Geometry check sheet. Reference: the model listing, model coordinates, mm. A direction names the side the tool comes from. Coordinates: 2 decimals unless noted, no trailing zeros. Loops run counter-clockwise (first coordinate to the right, second up) from the corner with the lowest first, then second, coordinate; pieces in that order, holes last. Notation, with made-up numbers: (-33.75, -10) -> (-19.75, -10) arc R18 ccw to (-19.75, 8) -> close; hole circle Ø11 at (-15, -10.5). An arc over 180 degrees is marked (long way). Answer as a JSON object with one key per item and string values.
from build123d import *

# Parameters (mm, degrees)
BOSS_EXTRU_1_DEPTH = 10
CONG_1_R           = 5


with BuildPart() as part:
    # Esquisse1 → Boss.-Extru.1 (new body)
    with BuildSketch(Plane.XY):
        Polygon((-20, 5), (20, 5), (50.310889132, 22.5), (90.310889132, 22.5), (90.310889132, 17.5), (50.310889132, 17.5), (20, 0), (-20, 0), align=None)
    extrude(amount=BOSS_EXTRU_1_DEPTH)

    # Congé1
    cong_1_edges = [part.edges().sort_by_distance(p)[0] for p in [
        (20, 0, 5),
        (50.310889132, 17.5, 5),
        (50.310889132, 22.5, 5),
        (20, 5, 5),
    ]]
    fillet(cong_1_edges, radius=CONG_1_R)


solid = part.part
1. Tool access check on faces 1 (the face through (-1, 5, 5)), 2 (the face through (-20, 2, 5)), 3 (the face through (71, 17.5, 5)). Record the directions out of +Z, -Z, +X, -X, +Y, -Y that give a thin tool (end or side, any length) a straight path to the whole face; none if there is none.
Evaluation:
{"face 1": "+Z, -Z, -X, +Y", "face 2": "+Z, -Z, -X, +Y, -Y", "face 3": "+Z, -Z, +X, -Y"}
2. Section check C-C, the plane y = 20. Record the boundary of the cut face in (x, z).
Evaluation:
{"outline": "(45.98, 0) -> (90.31, 0) -> (90.31, 10) -> (45.98, 10) -> close"}
3. Section check B-B, the plane x = 45. Record the boundary of the cut face in (y, z).
Evaluation:
{"outline": "(14.43, 0) -> (19.43, 0) -> (19.43, 10) -> (14.43, 10) -> close"}
4. Depth check by flat-ended pin: P1, Ø3, axis at x = 39.5, z = 9, coming from the +Y side; P2, Ø1, axis at x = 42, z = 2.5, coming from the +Y side; P3, Ø10, axis at x = 5.5, y = 12, coming from the -Z side; P4, Ø3, axis at y = 4, z = 2.5, coming from the +X side. Enter the tip coordinate at first touch or a pass-through.
Evaluation:
{"P1": "stops at y = 17.12", "P2": "stops at y = 17.99", "P3": "passes through", "P4": "stops at x = 29.53"}
5. Section check A-A, the plane z = 5.5. Record the boundary of the cut face in (x, y).
Evaluation:
{"outline": "(-20, 0) -> (18.66, 0) arc R5 ccw to (21.16, 0.67) -> (49.15, 16.83) arc R5 cw to (51.65, 17.5) -> (90.31, 17.5) -> (90.31, 22.5) -> (51.65, 22.5) arc R5 ccw to (49.15, 21.83) -> (21.16, 5.67) arc R5 cw to (18.66, 5) -> (-20, 5) -> close"}
6. Thickness scan on probe 1 along Y at (x, z) = (73, 0.5); probe 2 along Y at (x, z) = (17.5, 1.25); probe 3 along X at (y, z) = (17, 3). Record the ranges inside material, lowest first. Write a range as from..to.
Evaluation:
{"probe 1": "y = 17.5..22.5", "probe 2": "y = 0..5", "probe 3": "x = 40.78..49.47"}
